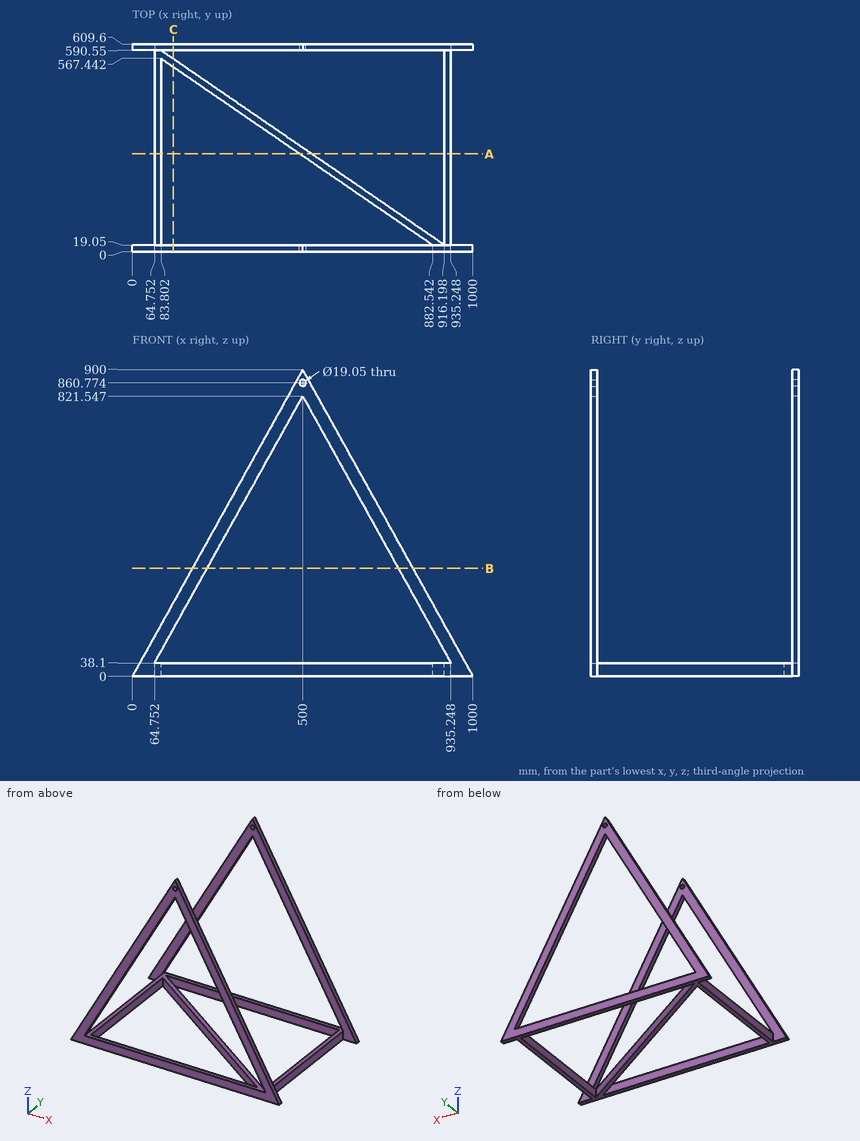
For this review, use the dimensioned drawing (mm, ordinates from the lowest corner) and the shaded views. Coordinates: 2 decimals unless noted, no trailing zeros. Loops run counter-clockwise (first coordinate to the right, second up) from the corner with the lowest first, then second, coordinate; pieces in that order, holes last.
1. Insertion check: P1, Ø11.5, axis at x = 500, z = 860.77, coming from the +Y side; P2, Ø11.5, axis at y = 283, z = 12.5, coming from the +X side; P3, Ø11.5, axis at y = 300, z = 22.5, coming from the -X side. Each pin has a flat end and moves straight along its axis. Give the tip position at first contact, or say it passes through.
2. For line 1 (Y direction, x = 607, z = 694), list the stretches that pass through material, from the lowest coordinate up.
3. Add section C-C, the plane x = 120. Give the boundary of the cut face in (y, z), then the cut area to 3 significant figures.
4. Add section A-A, the plane y = 287. Give the boundary of the cut face in (x, z) (1 decimal).
5. Add section B-B, the plane z = 316. Count the separate pieces of the cut face and the enclosed holes in it, then the cut area to 3 significant figures.
Result:
1. P1: passes through
1. P2: stops at x = 935.25
1. P3: stops at x = 64.75
2. line 1: y = 0 to 19.05, 590.55 to 609.6
3. outline: (0, 0) - (19.05, 0) - (19.05, 38.1) - (0, 38.1) - close; (0, 137.55) - (19.05, 137.55) - (19.05, 216) - (0, 216) - close; (542.59, 0) - (565.7, 0) - (565.7, 38.1) - (542.59, 38.1) - close; (590.55, 0) - (609.6, 0) - (609.6, 38.1) - (590.55, 38.1) - close; (590.55, 137.55) - (609.6, 137.55) - (609.6, 216) - (590.55, 216) - close
3. area: 5,320 mm2
4. outline: (64.8, 0) - (83.8, 0) - (83.8, 38.1) - (64.8, 38.1) - close; (492.3, 0) - (525.9, 0) - (525.9, 38.1) - (492.3, 38.1) - close; (916.2, 0) - (935.2, 0) - (935.2, 38.1) - (916.2, 38.1) - close
5. separate pieces: 4
5. enclosed holes: 0
5. area: 3,320 mm2
